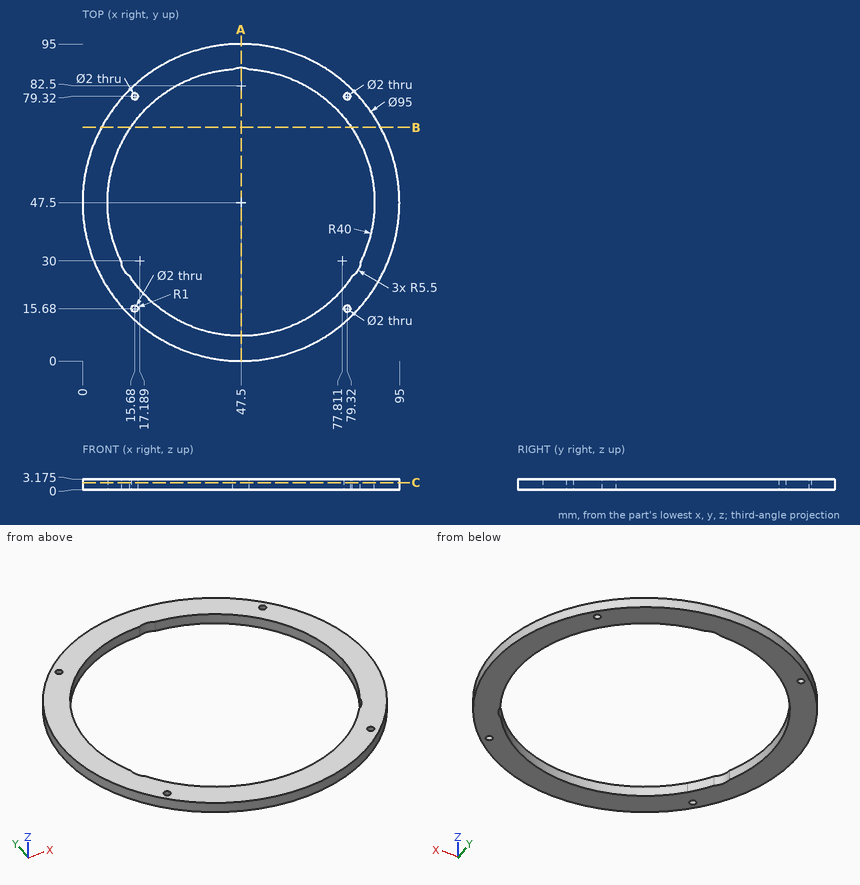
Verification items for this drawing (mm, ordinates from the low corner). Coordinates: 2 decimals unless noted, no trailing zeros. Write each loop counter-clockwise with the first axis right and the second up, starting at its lowest first coordinate (ties: lowest second). Pieces come first, ordered by that corner, then holes. Notation, with made-up numbers: (-38, 45) -> (6, 45) arc R30 ccw to (6, 69) -> close; hole circle Ø1 at (22, -36). An arc over 180 degrees is marked (long way). One line per item, written item: value. Start each with the question number.
Q1. Cross-section at C-C on z = 2.1. Enter the section's corners in (x, y) (1 decimal), and give its area (3 significant figures).
Q2. Cross-section at B-B on y = 70. Enter the section's corners in (x, z) (1 decimal).
Q3. Go/stop test with a flat-tipped pin: P1, Ø1.8, axis at x = 15.68, y = 15.68, coming from the -Z side. Record where the tip stops, or that it passes through.
Q4. Thickness scan on L1, parallel to X at y = 48.5, z = 0.75; L2, parallel to X at y = 78.5, z = 2.7; L3, parallel to X at y = 15.5, z = 0.4 (1 decimal). Record the ranges inside material, lowest first. Write a range as from..to.
Q5. Cross-section at A-A on x = 47.5. Enter the section's corners in (y, z) (3 decimals).
Checked values:
1. outline: circle Ø95 at (47.5, 47.5); hole (11.7, 29.7) arc R5.5 ccw to (14.1, 25.4) arc R40 ccw to (80.9, 25.4) arc R5.5 ccw to (83.3, 29.7) arc R40 ccw to (49.9, 87.4) arc R5.5 ccw to (45.1, 87.4) arc R40 ccw to start; hole circle Ø2 at (15.7, 15.7); hole circle Ø2 at (15.7, 79.3); hole circle Ø2 at (79.3, 15.7); hole circle Ø2 at (79.3, 79.3)
1. area: 2,040 mm²
2. outline: (5.7, 0) -> (14.4, 0) -> (14.4, 3.2) -> (5.7, 3.2) -> close; (80.6, 0) -> (89.3, 0) -> (89.3, 3.2) -> (80.6, 3.2) -> close
3. P1: passes through
4. L1: x = 0.01..7.51, 87.49..94.99
4. L2: x = 11.51..15.11, 16.25..22.22, 72.78..78.75, 79.89..83.49
4. L3: x = 12.4..14.7, 16.7..23.5, 71.5..78.3, 80.3..82.6
5. outline: (0, 0) -> (7.5, 0) -> (7.5, 3.175) -> (0, 3.175) -> close; (88, 0) -> (95, 0) -> (95, 3.175) -> (88, 3.175) -> close
